```python
from build123d import *

# Parameters (mm, degrees)
EXTRUDE_1_DEPTH     = 20
SKETCH_3_R          = 4.5
CUT_EXTRUDE_2_DEPTH = 20
CHAMFER_1_SIZE      = 5
CHAMFER_2_SIZE      = 5


with BuildPart() as part:
    # 草图1 → 凸台-拉伸1 (new body)
    with BuildSketch(Plane.XY):
        with BuildLine():
            Line((0, 5), (0, 30))
            Line((0, 30), (9.7, 30))
            Line((9.7, 30), (9.7, 21.3))
            ThreePointArc((9.7, 21.3), (13.975175508, 8.838258549), (25, 1.625397082))
            Line((25, 1.625397082), (25, 0))
            Line((25, 0), (6.25, 0))
            Line((6.25, 0), (0, 0))
            Line((0, 0), (0, -20))
            Line((0, -20), (-5, -20))
            Line((-5, -20), (-5, 5))
            Line((-5, 5), (0, 5))
        make_face()
    extrude(amount=EXTRUDE_1_DEPTH)

    # 草图3 → 切除-拉伸2 (cut)
    with BuildSketch(Plane.ZY.offset(5)):
        with Locations((10, -10)):
            Circle(SKETCH_3_R)
    extrude(amount=-CUT_EXTRUDE_2_DEPTH, mode=Mode.SUBTRACT)

    # 倒角1
    chamfer_1_edges = [part.edges().sort_by_distance(p)[0] for p in [
        (0, 5, 10),
    ]]
    chamfer(chamfer_1_edges, length=CHAMFER_1_SIZE - 0.0001)  # a hair under: the kernel refuses the full size

    # 倒角2
    chamfer_2_edges = [part.edges().sort_by_distance(p)[0] for p in [
        (0, 30, 10),
    ]]
    chamfer(chamfer_2_edges, length=CHAMFER_2_SIZE)


solid = part.part
```
Could you check a few things on this model? Use its own coordinates, in mm. A direction names the side the tool comes from. Give positions to 0.01 mm unless a question says otherwise; leave off trailing zeros. Order: outer loops, then holes, each group sorted by start corner. A loop starts at its lowest first (then second) coordinate and runs counter-clockwise, first axis right, second up.
Q1. I'm going to push flat-ended pins straight in: P1, Ø10, axis at x = 16.5, z = 13.5, coming from the -Y side; P2, Ø6, axis at y = 24, z = 16, coming from the -X side; P3, Ø6, axis at y = -9, z = 5.5, coming from the +X side. Where does each tip first touch, or does it pass through?
Q2. Suppose I cut it at B-B, the plane y = -10. Write out the boundary of the cut face in (x, z), and give its area (3 significant figures).
Q3. We'd pull the mould along Y, two halves only. Please class faces 1 (the flat face through (25, 1, 10)), 2 (the flat face through (3, 28, 10)), 3 (the cylindrical face through (-2.535, -8.648, 14.292)): +Y half, -Y half, draft (parallel to the pull), parting line (faces both ways), or undercut.
Q4. Suppose I cut it at D-D, the plane x = -0.5. Write out the boundary of the cut face in (y, z).
Q5. For faces 4 (the flat face through (0, 17, 10)), 5 (the flat face through (9.7, 26, 10)), 6 (the flat face through (13, 0, 10)), which set-ups out of +Z, -Z, +X, -X, +Y, -Y let a thin tool reach every point of the face, with its end or its side?
Q6. If I drill on line 1 along Y through (x, z) = (-2.55, 10); line 2 along Y through (x, z) = (-2.5, 11); line 3 along X through (y, z) = (-5, 18.25), over which ranges is the centre line in solid material (lowest first)?
Solution:
1. P1: stops at y = 0
1. P2: stops at x = 0
1. P3: stops at x = 0
2. outline: (-5, 0) - (0, 0) - (0, 5.5) - (-5, 5.5) - close; (-5, 14.5) - (0, 14.5) - (0, 20) - (-5, 20) - close
2. area: 55.0 mm2
3. face 1: draft
3. face 2: +Y half
3. face 3: undercut
4. outline: (-20, 0) - (9.5, 0) - (9.5, 20) - (-20, 20) - close; hole circle Ø9 at (-10, 10)
5. face 4: +Z, -Z, -X, +Y
5. face 5: +Z, -Z, +X, +Y
5. face 6: +Z, -Z, +X, -Y
6. line 1: y = -20 to -14.5, -5.5 to 7.45
6. line 2: y = -20 to -14.39, -5.61 to 7.5
6. line 3: x = -5 to 0
